Geometry check sheet. Reference: drawing and pictorial views, mm from the part's lowest x, y, z. Coordinates: 2 decimals unless noted, no trailing zeros. Loops run counter-clockwise (first coordinate to the right, second up) from the corner with the lowest first, then second, coordinate; pieces in that order, holes last. Notation, with made-up numbers: (44, 83) -> (78, 83) arc R23 ccw to (78, 109) -> close; hole circle Ø10 at (-30, -39). An arc over 180 degrees is marked (long way). Answer as a JSON object with one key per item and string values.
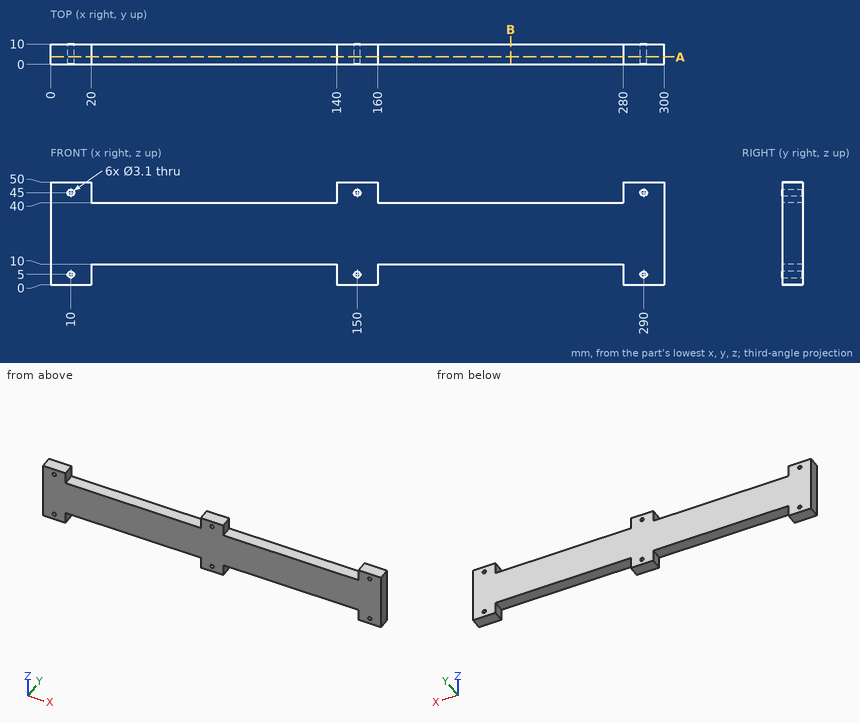
1. Thickness scan on probe 1 along X at (y, z) = (9.25, 43); probe 2 along X at (y, z) = (6, 45); probe 3 along Z at (x, y) = (150, 4). Record the ranges inside material, lowest first. Write a range as from..to.
Evaluation:
{"probe 1": "x = 0..20, 140..160, 280..300", "probe 2": "x = 0..8.45, 11.55..20, 140..148.45, 151.55..160, 280..288.45, 291.55..300", "probe 3": "z = 0..3.45, 6.55..43.45, 46.55..50"}
2. Section check B-B, the plane x = 225. Record the boundary of the cut face in (y, z).
Evaluation:
{"outline": "(0, 10) -> (10, 10) -> (10, 40) -> (0, 40) -> close"}
3. Section check A-A, the plane y = 3.75. Record the boundary of the cut face in (x, z).
Evaluation:
{"outline": "(0, 0) -> (20, 0) -> (20, 10) -> (140, 10) -> (140, 0) -> (160, 0) -> (160, 10) -> (280, 10) -> (280, 0) -> (300, 0) -> (300, 50) -> (280, 50) -> (280, 40) -> (160, 40) -> (160, 50) -> (140, 50) -> (140, 40) -> (20, 40) -> (20, 50) -> (0, 50) -> close; hole circle Ø3.1 at (10, 5); hole circle Ø3.1 at (10, 45); hole circle Ø3.1 at (150, 5); hole circle Ø3.1 at (150, 45); hole circle Ø3.1 at (290, 5); hole circle Ø3.1 at (290, 45)"}
4. Depth check by flat-ended pin: P1, Ø6, axis at y = 3, z = 35, coming from the -X side; P2, Ø3, axis at x = 107, y = 6, coming from the +Z side; P3, Ø5, axis at x = 70.5, y = 5, coming from the -Z side. Enter the tip coordinate at first touch or a pass-through.
Evaluation:
{"P1": "stops at x = 0", "P2": "stops at z = 40", "P3": "stops at z = 10"}
